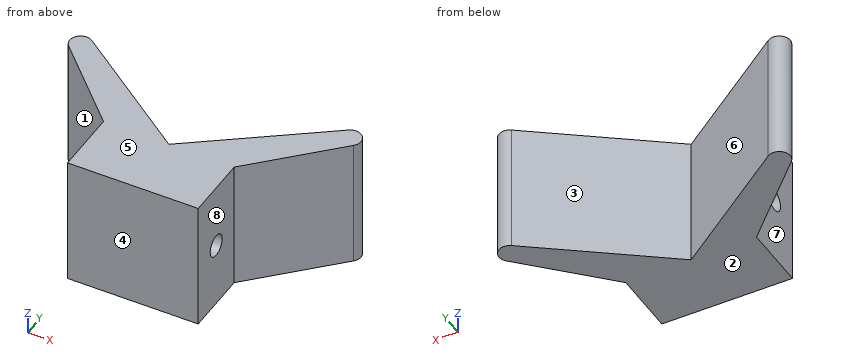
```python
from build123d import *

# Parameters (mm, degrees)
BOSS_EXTRUDE1_DEPTH = 76.2
SKETCH2_R           = 6.35
CUT_EXTRUDE1_DEPTH  = 123.988460527


with BuildPart() as part:
    # Sketch1 → Boss-Extrude1 (new body)
    with BuildSketch(Plane.XY):
        with BuildLine():
            Line((-38.1, 0), (38.1, 0))
            Line((38.1, 0), (38.1, 38.1))
            Line((38.1, 38.1), (83.018247276, 82.81205439))
            ThreePointArc((83.018247276, 82.81205439), (83.371778793, 91.430938362), (74.806024175, 92.449757914))
            Line((74.806024175, 92.449757914), (0, 38.1))
            Line((0, 38.1), (-74.806024175, 92.449757914))
            ThreePointArc((-74.806024175, 92.449757914), (-83.371778793, 91.430938362), (-83.018247276, 82.81205439))
            Line((-83.018247276, 82.81205439), (-38.1, 38.1))
            Line((-38.1, 38.1), (-38.1, 0))
        make_face()
    extrude(amount=BOSS_EXTRUDE1_DEPTH)

    # Sketch2 → Cut-Extrude1 (cut, through all)
    with BuildSketch(Plane(origin=(38.1, 0, 0), x_dir=(0, 0, -1), z_dir=(1, 0, 0))):
        with Locations((-38.1, 19.05)):
            Circle(SKETCH2_R)
    extrude(amount=-CUT_EXTRUDE1_DEPTH, mode=Mode.SUBTRACT)


solid = part.part
```
Build history of the part. All positions in model axes, mm. Face numbers are marked on the shaded views. A direction names the side the tool comes from. Give positions to 0.01 mm unless a question says otherwise; leave off trailing zeros. Loops run counter-clockwise (first coordinate to the right, second up) from the corner with the lowest first, then second, coordinate; pieces in that order, holes last.
1) Band-saw the part on C-C on z = 38.1. List the corners of the cut face in (x, y).
Values follow:
outline: (-83.02, 82.81) - (-38.1, 38.1) - (-38.1, 25.4) - (38.1, 25.4) - (38.1, 38.1) - (83.02, 82.81) arc R6.35 ccw to (74.81, 92.45) - (0, 38.1) - (-74.81, 92.45) arc R6.35 ccw to start; (-38.1, 0) - (38.1, 0) - (38.1, 12.7) - (-38.1, 12.7) - close
2) Two-plate mould, pull along X, no slides. Class the marked faces 1, 2 and 3: released by +X, released by -X, zero draft, split by the parting line, or undercut.
Values follow:
face 1: released by -X
face 2: zero draft
face 3: undercut
3) Band-saw the part on A-A on y = 19.05. List the corners of the cut face in (x, z), then the cut area to 3 significant figures.
Values follow:
outline: (-38.1, 0) - (38.1, 0) - (38.1, 31.75) - (-38.1, 31.75) - close; (-38.1, 44.45) - (38.1, 44.45) - (38.1, 76.2) - (-38.1, 76.2) - close
area: 4,840 mm2
4) 3-axis set-ups, long thin cutter, end or side, ignore diameter. For the marked faces 4, 5, 6, 7 and 8: which of +Z, -Z, +X, -X, +Y, -Y reach the whole face in a straight line?
Values follow:
face 4: +Z, -Z, +X, -X, -Y
face 5: +Z, +X, -X, +Y, -Y
face 6: +Z, -Z, +Y
face 7: +Z, -Z, -X, -Y
face 8: +Z, -Z, +X, -Y
5) Drop flat-ended pins along their axis: P1, Ø7.5, axis at y = 19.05, z = 38.1, coming from the +X side; P2, Ø1, axis at x = 45, z = 16.5, coming from the +Y side; P3, Ø8, axis at x = 11, z = 15, coming from the -Y side; P4, Ø2, axis at x = -57, z = 33, coming from the +Y side. Give the stop position or say it passes through.
Values follow:
P1: passes through
P2: stops at y = 71.16
P3: stops at y = 0
P4: stops at y = 80.24
6) Band-saw the part on B-B on z = 29. List the corners of the cut face in (x, y).
Values follow:
outline: (-83.02, 82.81) - (-38.1, 38.1) - (-38.1, 0) - (38.1, 0) - (38.1, 38.1) - (83.02, 82.81) arc R6.35 ccw to (74.81, 92.45) - (0, 38.1) - (-74.81, 92.45) arc R6.35 ccw to start
7) Probe line 1 along Z through (x, y) = (-9, 19); line 2 along Y through (x, z) = (5, 38); line 3 along X through (y, z) = (59.5, 10.5). List the from-to ranges inside material, lowest first.
Values follow:
line 1: z = 0 to 31.75, 44.45 to 76.2
line 2: y = 0 to 12.7, 25.4 to 41.73
line 3: x = -59.6 to -29.45, 29.45 to 59.6
8) Band-saw the part on D-D on x = -33. List the corners of the cut face in (y, z), then the cut area to 3 significant figures.
Values follow:
outline: (0, 0) - (62.08, 0) - (62.08, 76.2) - (0, 76.2) - close; hole circle Ø12.7 at (19.05, 38.1)
area: 4,600 mm2
